For this review, take the finished solid that the model builds, in its own axes (mm). A direction names the side the tool comes from. Round coordinates to 2 decimals unless told otherwise and drop trailing zeros. Order: outer loops, then holes, each group sorted by start corner. A loop starts at its lowest first (then second) coordinate and runs counter-clockwise, first axis right, second up. Notation, with made-up numbers: M -19.75,47.5 L 5.25,47.5 A23 cw 5.25,76.5 Z; hole C -25,7.5 d10. An arc over 180 degrees is marked long. Put each result on its own line as item: value.
from build123d import *

# Parameters (mm, degrees)
SKETCH_1_W               = 22.8
SKETCH_1_H               = 12.2
EXTRUDE_1_DEPTH          = 15.8
SKETCH_2_W               = 21
SKETCH_2_H               = 10.4
CUT_EXTRUDE_1_DEPTH      = 13.8
SKETCH_4_W               = 0.9
SKETCH_4_H               = 5.2
CUT_EXTRUDE_2_DEPTH      = 4
CUT_EXTRUDE_5_DEPTH      = 2
FILLET_2_R               = 0.5
SKETCH_8_W               = 0.9
SKETCH_8_H               = 5.2
CUT_EXTRUDE_6_DEPTH      = 4
EXTRUDE_2_DEPTH          = 13.8
CUT_EXTRUDE_8_DEPTH      = 19.91057905
CUT_EXTRUDE_8_DEPTH_BACK = 19.91057905
SKETCH_3_R               = 0.5
SKETCH_9_R               = 1.25
CUT_EXTRUDE_9_DEPTH      = 12
FILLET_3_R               = 0.5


with BuildPart() as part:
    # 草图1 → 凸台-拉伸1 (new body)
    with BuildSketch(Plane.XY):
        Rectangle(SKETCH_1_W, SKETCH_1_H)
    extrude(amount=EXTRUDE_1_DEPTH)

    # 草图2 → 切除-拉伸1 (cut)
    with BuildSketch(Plane.XY.offset(15.8)):
        Rectangle(SKETCH_2_W, SKETCH_2_H)
    extrude(amount=-CUT_EXTRUDE_1_DEPTH, mode=Mode.SUBTRACT)

    # 草图4 → 切除-拉伸2 (cut)
    with BuildSketch(Plane.XY.offset(15.8)):
        with Locations((-10.95, 0)):
            Rectangle(SKETCH_4_W, SKETCH_4_H)
    extrude(amount=-CUT_EXTRUDE_2_DEPTH, mode=Mode.SUBTRACT)

    # 草图7 → 切除-拉伸5 (cut)
    with BuildSketch(Plane.XY.offset(2)):
        with BuildLine():
            Line((-5.85, -0.2), (5.15, -0.2))
            ThreePointArc((5.15, -0.2), (7.4, -2.45), (5.15, -4.7))
            Line((5.15, -4.7), (-5.85, -4.7))
            ThreePointArc((-5.85, -4.7), (-8.1, -2.45), (-5.85, -0.2))
        make_face()
    extrude(amount=-CUT_EXTRUDE_5_DEPTH, mode=Mode.SUBTRACT)

    # 圆角2
    fillet_2_edges = [part.edges().sort_by_distance(p)[0] for p in [
        (11.4, -6.1, 7.9),
        (-11.4, -6.1, 7.9),
        (-11.4, 6.1, 7.9),
        (11.4, 6.1, 7.9),
    ]]
    fillet(fillet_2_edges, radius=FILLET_2_R)

    # 草图8 → 切除-拉伸6 (cut)
    with BuildSketch(Plane.XY.offset(15.8)):
        with Locations((10.95, 0)):
            Rectangle(SKETCH_8_W, SKETCH_8_H)
    extrude(amount=-CUT_EXTRUDE_6_DEPTH, mode=Mode.SUBTRACT)

    # 草图10 → 凸台-拉伸2 (add)
    with BuildSketch(Plane.XY.offset(2)):
        Polygon((-10.5, 3.2), (-10.5, 5.2), (-8.5, 5.2), align=None)
        Polygon((8.5, 5.2), (10.5, 5.2), (10.5, 3.2), align=None)
        Polygon((10.5, -3.2), (10.5, -5.2), (8.5, -5.2), align=None)
        Polygon((-10.5, -3.2), (-10.5, -5.2), (-8.5, -5.2), align=None)
    extrude(amount=EXTRUDE_2_DEPTH)

    # 草图3 → 切除-拉伸8 (cut, two sides: drawn at the far end of the back side and taken through both)
    with BuildSketch(Plane.XY.offset(2).offset(-CUT_EXTRUDE_8_DEPTH_BACK)):
        with Locations((9.9, 4.6)):
            Circle(SKETCH_3_R)
        with Locations((-9.9, -4.6)):
            Circle(SKETCH_3_R)
        with Locations((9.9, -4.6)):
            Circle(SKETCH_3_R)
        with Locations((-9.9, 4.6)):
            Circle(SKETCH_3_R)
    extrude(amount=CUT_EXTRUDE_8_DEPTH + CUT_EXTRUDE_8_DEPTH_BACK, mode=Mode.SUBTRACT)

    # 草图9 → 切除-拉伸9 (cut)
    with BuildSketch(Plane(origin=(0, 0, 0), x_dir=(-1, 0, 0), z_dir=(0, 0, -1))):
        with Locations((-9.9, 4.6)):
            Circle(SKETCH_9_R)
        with Locations((9.9, 4.6)):
            Circle(SKETCH_9_R)
        with Locations((-9.9, -4.6)):
            Circle(SKETCH_9_R)
        with Locations((9.9, -4.6)):
            Circle(SKETCH_9_R)
    extrude(amount=-CUT_EXTRUDE_9_DEPTH, mode=Mode.SUBTRACT)

    # 圆角3
    # the kernel refuses this fillet: 0.5 mm, written as the material it takes off along each edge
    with BuildSketch(Plane(origin=(-10.9, 6.1, 0), x_dir=(0, 0, 1), z_dir=(1, 0, 0))) as fillet_3_piece_1:
        with BuildLine():
            CenterArc((FILLET_3_R, FILLET_3_R), FILLET_3_R, 180, 90)
            Line((0, FILLET_3_R), (0, 0))
            Line((0, 0), (FILLET_3_R, 0))
        make_face()
    extrude(amount=21.8, mode=Mode.SUBTRACT)
    with BuildSketch(Plane(origin=(11.4, 5.6, 0), x_dir=(-1, 0, 0), z_dir=(0, -1, 0)), Plane(origin=(-11.4, -5.6, 0), x_dir=(1, 0, 0), z_dir=(0, 1, 0))) as fillet_3_piece_2:
        with BuildLine():
            CenterArc((FILLET_3_R, -FILLET_3_R), FILLET_3_R, 90, 90)
            Line((0, -FILLET_3_R), (0, 0))
            Line((0, 0), (FILLET_3_R, 0))
        make_face()
    extrude(amount=11.2, mode=Mode.SUBTRACT)
    with BuildSketch(Plane(origin=(10.9, -6.1, 0), x_dir=(0, 1, 0), z_dir=(-1, 0, 0))) as fillet_3_piece_3:
        with BuildLine():
            CenterArc((FILLET_3_R, -FILLET_3_R), FILLET_3_R, 90, 90)
            Line((0, -FILLET_3_R), (0, 0))
            Line((0, 0), (FILLET_3_R, 0))
        make_face()
    extrude(amount=21.8, mode=Mode.SUBTRACT)
    with BuildSketch(Plane(origin=(-10.9, 5.6, 0), x_dir=(0, 1, 0), z_dir=(1, 0, 0))) as fillet_3_piece_4:
        with BuildLine():
            CenterArc((0.5 - FILLET_3_R, FILLET_3_R), FILLET_3_R, 270, 90)
            Line((0.5, FILLET_3_R), (0.5, 0))
            Line((0.5, 0), (0.5 - FILLET_3_R, 0))
        make_face()
    revolve(axis=Axis((-10.9, 5.6, 0), (0, 0, 1)), revolution_arc=90, mode=Mode.SUBTRACT)
    with BuildSketch(Plane(origin=(-10.9, -5.6, 0), x_dir=(-1, 0, 0), z_dir=(0, 1, 0))) as fillet_3_piece_5:
        with BuildLine():
            CenterArc((0.5 - FILLET_3_R, FILLET_3_R), FILLET_3_R, 270, 90)
            Line((0.5, FILLET_3_R), (0.5, 0))
            Line((0.5, 0), (0.5 - FILLET_3_R, 0))
        make_face()
    revolve(axis=Axis((-10.9, -5.6, 0), (0, 0, 1)), revolution_arc=90, mode=Mode.SUBTRACT)
    with BuildSketch(Plane(origin=(10.9, -5.6, 0), x_dir=(1, 0, 0), z_dir=(0, 1, 0))) as fillet_3_piece_6:
        with BuildLine():
            CenterArc((0.5 - FILLET_3_R, -FILLET_3_R), FILLET_3_R, 0, 90)
            Line((0.5, -FILLET_3_R), (0.5, 0))
            Line((0.5, 0), (0.5 - FILLET_3_R, 0))
        make_face()
    revolve(axis=Axis((10.9, -5.6, 0), (0, 0, -1)), revolution_arc=90, mode=Mode.SUBTRACT)
    with BuildSketch(Plane(origin=(10.9, 5.6, 0), x_dir=(0, 1, 0), z_dir=(-1, 0, 0))) as fillet_3_piece_7:
        with BuildLine():
            CenterArc((0.5 - FILLET_3_R, -FILLET_3_R), FILLET_3_R, 0, 90)
            Line((0.5, -FILLET_3_R), (0.5, 0))
            Line((0.5, 0), (0.5 - FILLET_3_R, 0))
        make_face()
    revolve(axis=Axis((10.9, 5.6, 0), (0, 0, -1)), revolution_arc=90, mode=Mode.SUBTRACT)


solid = part.part
(1) Add section D-D on y = -2. Give the boundary of the cut face in (x, z).
A:
outline: M -11.4,0.5 A0.5 ccw -10.9,0 L -8.05,0 L -8.05,2 L -10.5,2 L -10.5,11.8 L -11.4,11.8 Z; M 7.35,0 L 10.9,0 A0.5 ccw 11.4,0.5 L 11.4,11.8 L 10.5,11.8 L 10.5,2 L 7.35,2 Z
(2) Add section B-B on x = -5.25. Give the boundary of the cut face in (y, z), then the cut area to 3 significant figures.
A:
outline: M -6.1,0.5 A0.5 ccw -5.6,0 L -4.7,0 L -4.7,2 L -5.2,2 L -5.2,15.8 L -6.1,15.8 Z; M -0.2,0 L 5.6,0 A0.5 ccw 6.1,0.5 L 6.1,15.8 L 5.2,15.8 L 5.2,2 L -0.2,2 Z
area: 40.1 mm2
(3) Draft analysis for pull direction X (two halves, no side actions). For faces 4 (the face through (7.4, -2.4, 1)), 5 (the face through (11.4, 0, 8)), 6 (the face through (-0.1, -5.6, 15.8)), state which applies: released by +X, released by -X, zero draft, split by the parting line, or undercut.
A:
face 4: undercut
face 5: released by +X
face 6: zero draft
(4) Add section C-C on y = 4.6. Give the boundary of the cut face in (x, z), then the cut area to 3 significant figures.
A:
outline: M -11.4,0.5 A0.5 ccw -11.15,0.07 L -11.15,12 L -10.4,12 L -10.4,15.8 L -11.4,15.8 Z; M -9.4,12 L -9.1,12 L -9.1,15.8 L -9.4,15.8 Z; M -8.65,0 L 8.65,0 L 8.65,2 L -8.65,2 Z; M 9.1,12 L 9.4,12 L 9.4,15.8 L 9.1,15.8 Z; M 10.4,12 L 11.15,12 L 11.15,0.07 A0.5 ccw 11.4,0.5 L 11.4,15.8 L 10.4,15.8 Z
area: 50.4 mm2
(5) For faces 1 (the face through (-10.2, -5.2, 12)), 2 (the face through (11, -2.6, 14)), 3 (the face through (0, 5.2, 9)), list the 3-axis set-ups (+Z, -Z, +X, -X, +Y, -Y) from which the entire face can be reached by the end or side of a thin tool; tool diameter is ignored.
A:
face 1: -Z
face 2: +Z, +X, -X
face 3: +Z
(6) Insertion check: pin 1 Ø1 at (x, y) = (11, -1) entering from +Z. The pin has a flat end and moves straight along its axis. Give the tip position at first contact, or say it passes through.
A:
pin 1: stops at z = 11.8
(7) Add section A-A on z = 14.25. Give the boundary of the cut face in (x, y).
A:
outline: M -11.4,-5.6 A0.5 ccw -10.9,-6.1 L 10.9,-6.1 A0.5 ccw 11.4,-5.6 L 11.4,-2.6 L 10.5,-2.6 L 10.5,-3.2 L 8.5,-5.2 L -8.5,-5.2 L -10.5,-3.2 L -10.5,-2.6 L -11.4,-2.6 Z; M -11.4,2.6 L -10.5,2.6 L -10.5,3.2 L -8.5,5.2 L 8.5,5.2 L 10.5,3.2 L 10.5,2.6 L 11.4,2.6 L 11.4,5.6 A0.5 ccw 10.9,6.1 L -10.9,6.1 A0.5 ccw -11.4,5.6 Z; hole C -9.9,-4.6 d1; hole C -9.9,4.6 d1; hole C 9.9,-4.6 d1; hole C 9.9,4.6 d1
(8) To check wall thickness, follow L1, parallel to Y at x = -3.5, z = 14.5; L2, parallel to Y at x = 9.9, z = 5; L3, parallel to X at y = 4.5, z = 13.75. State the ranges of each line that lie inside material, in increasing order.
A:
L1: y = -6.1 to -5.2, 5.2 to 6.1
L2: y = -6.1 to -5.85, 5.85 to 6.1
L3: x = -11.4 to -10.39, -9.41 to -9.2, 9.2 to 9.41, 10.39 to 11.4
